```python
from build123d import *

# Parameters (mm, degrees)
F0_R     = 52.5
F1_DEPTH = 10
F2_R     = 22.5
F2_R_2   = 16
F3_DEPTH = 5
F4_R     = 22.5
F4_R_2   = 16
F5_DEPTH = 4.5
F6_R     = 16
F7_DEPTH = 25


with BuildPart() as f1:
    # F0 (on Front) → F1 (new body)
    with BuildSketch(Plane.XZ):
        Circle(F0_R)
        with BuildLine():
            ThreePointArc((4.9913419848, 42.2058823529), (30.0520382004, 30.0520382004), (42.2058823529, 4.9913419848))
            ThreePointArc((42.2058823529, 4.9913419848), (45.9299717029, 3.6380343755), (47.5, 0))
            ThreePointArc((47.5, 0), (45.9299717029, -3.6380343755), (42.2058823529, -4.9913419848))
            ThreePointArc((42.2058823529, -4.9913419848), (30.0520382004, -30.0520382004), (4.9913419848, -42.2058823529))
            ThreePointArc((4.9913419848, -42.2058823529), (4.9978350275, -42.3528774732), (5, -42.5))
            ThreePointArc((5, -42.5), (-0.1471225268, -47.4978350275), (-4.9913419848, -42.2058823529))
            ThreePointArc((-4.9913419848, -42.2058823529), (-30.0520382004, -30.0520382004), (-42.2058823529, -4.9913419848))
            ThreePointArc((-42.2058823529, -4.9913419848), (-47.5, 0), (-42.2058823529, 4.9913419848))
            ThreePointArc((-42.2058823529, 4.9913419848), (-30.0520382004, 30.0520382004), (-4.9913419848, 42.2058823529))
            ThreePointArc((-4.9913419848, 42.2058823529), (-0.1471225268, 47.4978350275), (5, 42.5))
            ThreePointArc((5, 42.5), (4.9978350275, 42.3528774732), (4.9913419848, 42.2058823529))
        make_face(mode=Mode.SUBTRACT)
        with BuildLine():
            ThreePointArc((42.2058823529, -4.9913419848), (37.5, 0), (42.2058823529, 4.9913419848))
            ThreePointArc((42.2058823529, 4.9913419848), (30.0520382004, 30.0520382004), (4.9913419848, 42.2058823529))
            ThreePointArc((4.9913419848, 42.2058823529), (0, 37.5), (-4.9913419848, 42.2058823529))
            ThreePointArc((-4.9913419848, 42.2058823529), (-30.0520382004, 30.0520382004), (-42.2058823529, 4.9913419848))
            ThreePointArc((-42.2058823529, 4.9913419848), (-38.8619656245, 3.4299717029), (-37.5, 0))
            ThreePointArc((-37.5, 0), (-38.8619656245, -3.4299717029), (-42.2058823529, -4.9913419848))
            ThreePointArc((-42.2058823529, -4.9913419848), (-30.0520382004, -30.0520382004), (-4.9913419848, -42.2058823529))
            ThreePointArc((-4.9913419848, -42.2058823529), (0, -37.5), (4.9913419848, -42.2058823529))
            ThreePointArc((4.9913419848, -42.2058823529), (30.0520382004, -30.0520382004), (42.2058823529, -4.9913419848))
        make_face()
    extrude(amount=F1_DEPTH)

    # F2 (on face) → F3 (cut)
    with BuildSketch(Plane.XZ.offset(10)):
        Circle(F2_R)
        Circle(F2_R_2, mode=Mode.SUBTRACT)
        Circle(F2_R_2)
    extrude(amount=-F3_DEPTH, mode=Mode.SUBTRACT)

    # F4 (on face) → F5 (join)
    with BuildSketch(Plane(origin=(0, 0, 0), x_dir=(-1, 0, 0), z_dir=(0, 1, 0))):
        Circle(F4_R)
        Circle(F4_R_2, mode=Mode.SUBTRACT)
    extrude(amount=F5_DEPTH)

    # F6 (on face) → F7 (cut)
    with BuildSketch(Plane(origin=(0, 0, 0), x_dir=(-1, 0, 0), z_dir=(0, 1, 0))):
        Circle(F6_R)
    extrude(amount=-F7_DEPTH, mode=Mode.SUBTRACT)


solid = f1.part
```
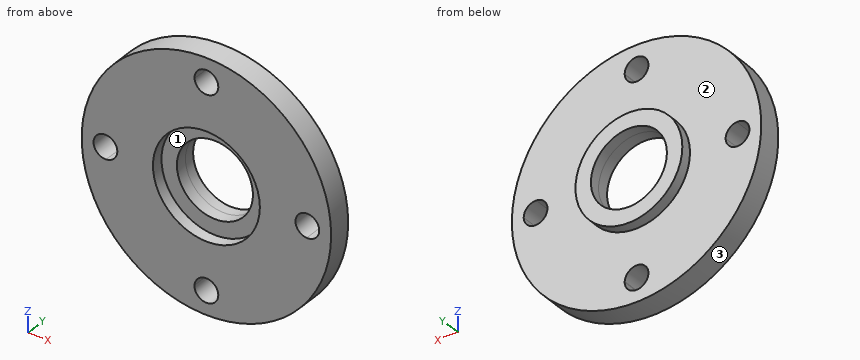
Model file for the job. Use its own axes, mm. Face numbers are marked on the shaded views. Round coordinates to 2 decimals unless told otherwise and drop trailing zeros. Write each loop counter-clockwise with the first axis right and the second up, starting at its lowest first coordinate (ties: lowest second). Pieces come first, ordered by that corner, then holes. Notation, with made-up numbers: (46, 73) - (64, 73) arc R24 cw to (64, 107) - close; hole circle Ø2 at (-25.5, 52). An arc over 180 degrees is marked (long way). Use CSV: the item, a comma, the result in double quotes. Start each with the question number.
Item 1: Band-saw the part on A-A (x = 0). Write the cut outline in (y, z).
Item 2: Pin check, flat tips, straight feed: P1, Ø8, axis at x = 24, y = -3, coming from the -Z side; P2, Ø2, axis at y = -5.5, z = 39.5, coming from the -X side; P3, Ø4, axis at x = -28.5, y = -3, coming from the -Z side. Stop position of each tip, or through.
Item 3: Band-saw the part on B-B (y = -1.25). Write the cut outline in (x, z).
Item 4: Band-saw the part on C-C (x = 43.5). Write the cut outline in (y, z).
Item 5: Two-plate mould, pull along X, no slides. Class the marked faces 1, 2 and 3: released by +X, released by -X, zero draft, split by the parting line, or undercut.
Item 6: Band-saw the part on D-D (y = -7.25). Write the cut outline in (x, z).
Item 7: Drill centre lines: L1, parallel to Z at x = 0, y = -1.95; L2, parallel to Z at x = 0, y = 1; L3, parallel to X at y = -6.75, z = -7.5. Where is each one in solid material? Low to high. Write a range as [from, to].
Checked values:
1,outline,"(-10, -52.5) - (0, -52.5) - (0, -47.5) - (-10, -47.5) - close; (-10, -37.5) - (0, -37.5) - (0, -22.5) - (4.5, -22.5) - (4.5, -16) - (-5, -16) - (-5, -22.5) - (-10, -22.5) - close; (-10, 22.5) - (-5, 22.5) - (-5, 16) - (4.5, 16) - (4.5, 22.5) - (0, 22.5) - (0, 37.5) - (-10, 37.5) - close; (-10, 47.5) - (0, 47.5) - (0, 52.5) - (-10, 52.5) - close"
2,P1,"stops at z = -48.54"
2,P2,"stops at x = -35.69"
2,P3,"stops at z = -45.32"
3,outline,"circle Ø105 at (0, 0); hole circle Ø10 at (-42.5, 0); hole circle Ø32 at (0, 0); hole circle Ø10 at (0, -42.5); hole circle Ø10 at (0, 42.5); hole circle Ø10 at (42.5, 0)"
4,outline,"(-10, -29.39) - (0, -29.39) - (0, -4.9) - (-10, -4.9) - close; (-10, 4.9) - (0, 4.9) - (0, 29.39) - (-10, 29.39) - close"
5,face 1,"undercut"
5,face 2,"zero draft"
5,face 3,"split by the parting line"
6,outline,"circle Ø105 at (0, 0); hole circle Ø10 at (-42.5, 0); hole circle Ø45 at (0, 0); hole circle Ø10 at (0, -42.5); hole circle Ø10 at (0, 42.5); hole circle Ø10 at (42.5, 0)"
7,L1,"z = [-52.5, -47.5], [-37.5, -16], [16, 37.5], [47.5, 52.5]"
7,L2,"z = [-22.5, -16], [16, 22.5]"
7,L3,"x = [-51.96, -21.21], [21.21, 51.96]"
